Read the model definition and answer for the solid it produces. Units are mm, in the model's axes. Face numbers are marked on the shaded views. A direction names the side the tool comes from. Round coordinates to 2 decimals unless told otherwise and drop trailing zeros. Loops run counter-clockwise (first coordinate to the right, second up) from the corner with the lowest first, then second, coordinate; pieces in that order, holes last. Notation, with made-up numbers: (58.25, 64) -> (65.25, 64) arc R28 cw to (65.25, 83) -> close; hole circle Ø5 at (64, -10). An arc over 180 degrees is marked (long way). Put each result on its own line as item: value.
from build123d import *

# Parameters (mm, degrees)
BOSS_EXTRUDE1_DEPTH = 30
SKETCH4_W           = 22
SKETCH4_H           = 10
CUT_EXTRUDE2_DEPTH  = 15
SKETCH5_W           = 1.5
SKETCH5_H           = 1.8
CUT_EXTRUDE3_DEPTH  = 15
CUT_EXTRUDE4_DEPTH  = 11
SKETCH7_R           = 1.2
CUT_EXTRUDE5_DEPTH  = 4


with BuildPart() as part:
    # Sketch1 → Boss-Extrude1 (new body)
    with BuildSketch(Plane.XY):
        Polygon((0, 0), (0, -25), (12, -25), (12, -18), (4, 0), align=None)
    extrude(amount=-BOSS_EXTRUDE1_DEPTH)

    # Sketch4 → Cut-Extrude2 (cut)
    with BuildSketch(Plane.ZY):
        with Locations((-16, -20.207997185)):
            Rectangle(SKETCH4_W, SKETCH4_H)
    extrude(amount=-CUT_EXTRUDE2_DEPTH, mode=Mode.SUBTRACT)

    # Sketch5 → Cut-Extrude3 (cut)
    with BuildSketch(Plane.ZY):
        with Locations((-4.25, -22.7)):
            Rectangle(SKETCH5_W, SKETCH5_H)
    cut_extrude3 = extrude(amount=-CUT_EXTRUDE3_DEPTH, mode=Mode.SUBTRACT)

    # Mirror1: Cut-Extrude3 across plane
    add(cut_extrude3.mirror(Plane.XY.offset(-16)), mode=Mode.SUBTRACT)

    # Sketch6 → Cut-Extrude4 (cut, symmetric)
    with BuildSketch(Plane.XY.offset(-16)):
        Polygon((4, 0), (4, -13), (9.777777778, -13), align=None)
    extrude(amount=CUT_EXTRUDE4_DEPTH, both=True, mode=Mode.SUBTRACT)

    # Sketch7 → Cut-Extrude5 (cut)
    with BuildSketch(Plane(origin=(0, -13, 0), x_dir=(1, 0, 0), z_dir=(0, 1, 0))):
        with Locations(Location((6.172753197, 16, 0), (0, 0, 270))):
            Circle(SKETCH7_R)
    extrude(amount=-CUT_EXTRUDE5_DEPTH, mode=Mode.SUBTRACT)


solid = part.part
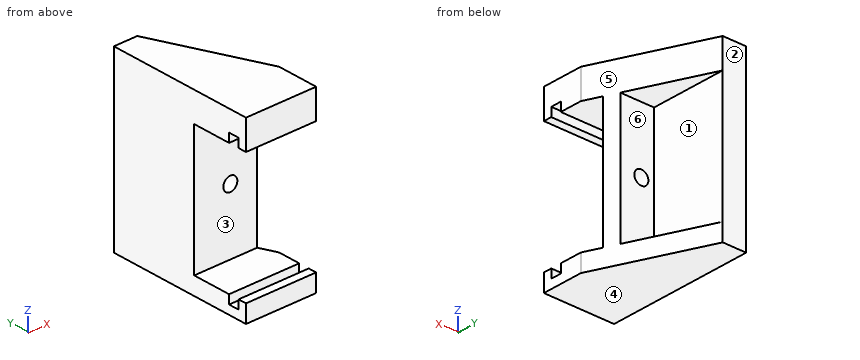
Item 1: The part is cut by section B-B (z = -16). Determine the outline of the cut face in (x, y), then the cut area to 3 significant figures.
Derived:
outline: (0, -15.21) -> (4.97, -15.21) -> (4.97, -13) -> (4, -13) -> (4, 0) -> (0, 0) -> close; (7.37, -15.21) -> (10.76, -15.21) -> (9.78, -13) -> (7.37, -13) -> close
area: 69.4 mm^2
Item 2: The part is cut by section A-A (y = -20.5). Determine the outline of the cut face in (x, z), then the cut area to 3 significant figures.
Derived:
outline: (0, -30) -> (12, -30) -> (12, -27) -> (0, -27) -> close; (0, -5) -> (12, -5) -> (12, 0) -> (0, 0) -> close
area: 96.0 mm^2
Item 3: The part is cut by section C-C (x = 2.5). Determine the outline of the cut face in (y, z).
Derived:
outline: (-25, -30) -> (0, -30) -> (0, 0) -> (-25, 0) -> (-25, -5) -> (-23.6, -5) -> (-23.6, -3.5) -> (-21.8, -3.5) -> (-21.8, -5) -> (-15.21, -5) -> (-15.21, -27) -> (-21.8, -27) -> (-21.8, -28.5) -> (-23.6, -28.5) -> (-23.6, -27) -> (-25, -27) -> close
Item 4: For a pull along Z with two mould halves and no side action, classify the marked faces 4, 5 and 6 as pulls with the +Z half, pulls with the -Z half, needs draft (parallel to the pull), parting line crosses it, or undercut.
Derived:
face 4: pulls with the -Z half
face 5: needs draft
face 6: undercut
Item 5: Flat-ended cylindrical pins translate along their axes: pin 1 Ø3 at (x, z) = (7.5, -14) entering from -Y; pin 2 Ø4 at (y, z) = (-9.5, -18.5) entering from +X. Find the tip coordinate at first contact, or state that the pin passes through.
Derived:
pin 1: stops at y = -15.21
pin 2: stops at x = 4
Item 6: Find the intervals of material crossed by line 1 along Z through (x, y) = (1.5, -16.5); line 2 along Y through (x, z) = (0.5, -4.75); line 3 along Y through (x, z) = (8, -26), in increasing order.
Derived:
line 1: z = -30 to -27, -5 to 0
line 2: y = -25 to -23.6, -21.8 to 0
line 3: y = -15.21 to -13
Item 7: Which of the six approach directions +Z, -Z, +X, -X, +Y, -Y give full straight-line access (tool end or side, diameter ignored) to the marked faces 1, 2 and 3?
Derived:
face 1: +X, +Y
face 2: +Z, -Z, +X, -X, +Y
face 3: +X, -X, -Y
Item 8: The part is cut by section D-D (z = -19.25). Determine the outline of the cut face in (x, y).
Derived:
outline: (0, -15.21) -> (10.76, -15.21) -> (9.78, -13) -> (4, -13) -> (4, 0) -> (0, 0) -> close
